Design review of the part shown in the three views and the two pictorial views. Dimensions are in mm from the part's minimum x, y and z. A direction names the side the tool comes from. Coordinates: 2 decimals unless noted, no trailing zeros. Write each loop counter-clockwise with the first axis right and the second up, starting at its lowest first coordinate (ties: lowest second). Pieces come first, ordered by that corner, then holes.
Q1. Take a section at C-C, the plane z = 26. Write out the cut boundary in (x, y), plus the area to 3 significant figures.
Q2. Take a section at B-B, the plane y = 25. Write out the cut boundary in (x, z), plus the area to 3 significant figures.
Q3. Take a section at A-A, the plane x = 25. Write out the cut boundary in (y, z).
Q4. For L1, parallel to Y at x = 25, z = 116.5; L2, parallel to Y at x = 25, z = 41; L3, parallel to Y at x = 38.5, z = 105, list the stretches that pass through material, from the lowest coordinate up.
Q5. The part is to be moulded in two halves that separate along Y. For the marked faces 1 and 2, say which applies: released by +Y, released by -Y, zero draft, split by the parting line, or undercut.
Q6. For the marked faces 3, 4 and 5, list the 3-axis set-ups (+Z, -Z, +X, -X, +Y, -Y) from which the entire face can be reached by the end or side of a thin tool; tool diameter is ignored.
Q7. For pin 1 Ø3 at (x, z) = (12, 16.5) entering from +Y; pin 2 Ø5 at (x, y) = (17, 65) entering from +Z; pin 3 Ø4 at (y, z) = (53, 80) entering from +X, all flat-tipped, find the tip position at first contact; note any pin that passes through.
Q8. Take a section at D-D, the plane y = 97.5. Write out the cut boundary in (x, z).
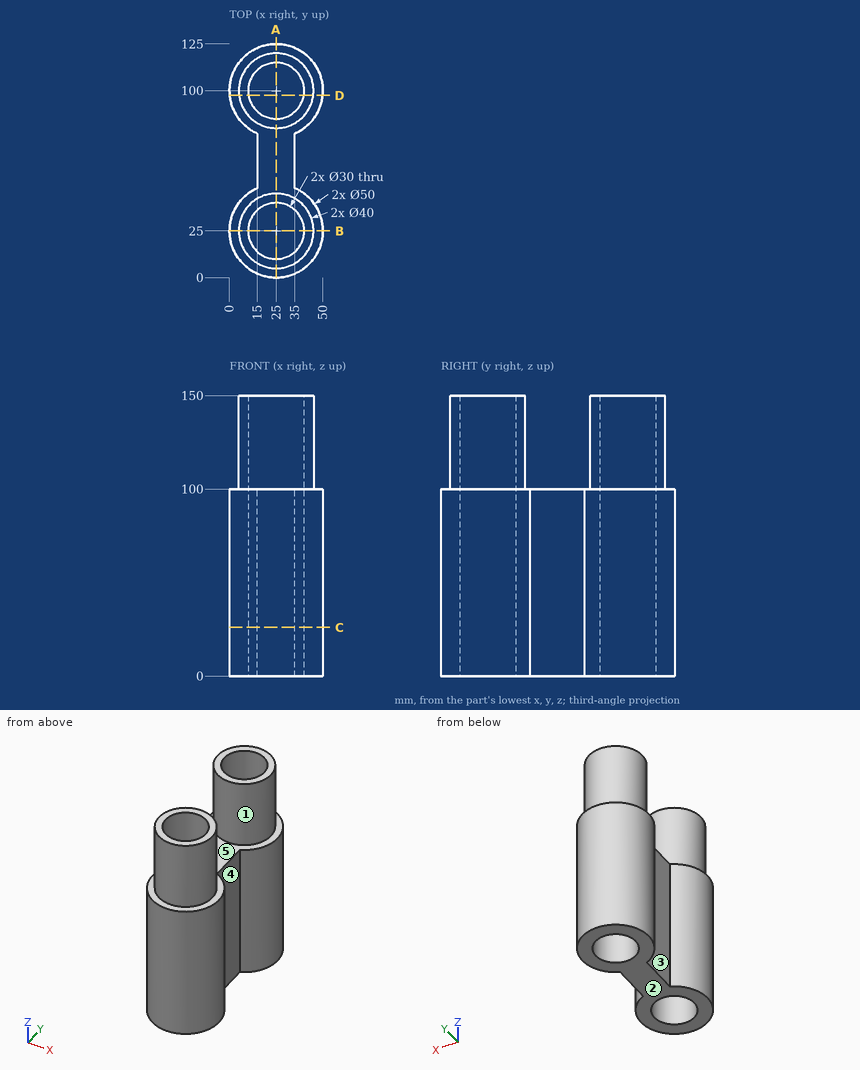
Responses:
1. outline: (15, 47.91) arc R25 ccw (long way) to (35, 47.91) - (35, 77.09) arc R25 ccw (long way) to (15, 77.09) - close; hole circle Ø30 at (25, 25); hole circle Ø30 at (25, 100)
1. area: 3,040 mm2
2. outline: (0, 0) - (10, 0) - (10, 150) - (5, 150) - (5, 100) - (0, 100) - close; (40, 0) - (50, 0) - (50, 100) - (45, 100) - (45, 150) - (40, 150) - close
2. area: 2,500 mm2
3. outline: (0, 0) - (10, 0) - (10, 150) - (5, 150) - (5, 100) - (0, 100) - close; (40, 0) - (85, 0) - (85, 150) - (80, 150) - (80, 100) - (45, 100) - (45, 150) - (40, 150) - close; (115, 0) - (125, 0) - (125, 100) - (120, 100) - (120, 150) - (115, 150) - close
4. L1: y = 5 to 10, 40 to 45, 80 to 85, 115 to 120
4. L2: y = 0 to 10, 40 to 85, 115 to 125
4. L3: y = 10.24 to 18.46, 31.54 to 39.76, 85.24 to 93.46, 106.54 to 114.76
5. face 1: undercut
5. face 2: zero draft
6. face 3: +Z, -Z, -X
6. face 4: +Z, -Z, +X
6. face 5: +Z
7. pin 1: stops at y = 122.2
7. pin 2: stops at z = 100
7. pin 3: stops at x = 35
8. outline: (0.13, 0) - (10.21, 0) - (10.21, 150) - (5.16, 150) - (5.16, 100) - (0.13, 100) - close; (39.79, 0) - (49.87, 0) - (49.87, 100) - (44.84, 100) - (44.84, 150) - (39.79, 150) - close
